Here's how the part is built. I have some questions about the finished solid (model axes, mm). A direction names the side the tool comes from. Give positions to 0.01 mm unless a question says otherwise; leave off trailing zeros. Order: outer loops, then holes, each group sorted by start corner. A loop starts at its lowest first (then second) coordinate and runs counter-clockwise, first axis right, second up.
from build123d import *

# Parameters (mm, degrees)
SKETCH1_R                  = 6
BOSS_EXTRUDE1_DEPTH        = 22
SKETCH2_R                  = 6
BOSS_EXTRUDE2_DEPTH        = 10
BOSS_EXTRUDE3_START        = -8
SKETCH3_R                  = 6
BOSS_EXTRUDE3_DEPTH        = 8
M6X1_0_TAPPED_HOLE1_D      = 5
M6X1_0_TAPPED_HOLE1_DEPTH  = 16
M6X1_0_TAPPED_HOLE1_TIP    = 1.443375673
SKETCH6_R                  = 6
CUT_EXTRUDE1_DEPTH         = 4
M6X1_0_TAPPED_HOLE2_REACH  = 63.741
M6X1_0_TAPPED_HOLE2_BORE_R = 2.5


with BuildPart() as part:
    # Sketch1 → Boss-Extrude1 (new body)
    with BuildSketch(Plane.XY):
        with BuildLine():
            Line((-8, 0), (8, 0))
            Line((8, 0), (8, 10))
            Line((8, 10), (32, 10))
            Line((32, 10), (32, 20))
            Line((32, 20), (24.228334067, 20))
            ThreePointArc((24.228334067, 20), (22.616435242, 20.469825663), (21.509410706, 21.732145215))
            Line((21.509410706, 21.732145215), (14.500924593, 36.761892188))
            ThreePointArc((14.500924593, 36.761892188), (0, 46), (-14.500924593, 36.761892188))
            Line((-14.500924593, 36.761892188), (-21.509410706, 21.732145215))
            ThreePointArc((-21.509410706, 21.732145215), (-22.616435242, 20.469825663), (-24.228334067, 20))
            Line((-24.228334067, 20), (-32, 20))
            Line((-32, 20), (-32, 10))
            Line((-32, 10), (-8, 10))
            Line((-8, 10), (-8, 0))
        make_face()
        with Locations((0, 30)):
            Circle(SKETCH1_R, mode=Mode.SUBTRACT)
    extrude(amount=-BOSS_EXTRUDE1_DEPTH)

    # Sketch2 → Boss-Extrude2 (add)
    with BuildSketch(Plane(origin=(0, 0, -22), x_dir=(-1, 0, 0), z_dir=(0, 0, -1))):
        Polygon((-32, 10), (-32, 46), (32, 46), (32, 10), (8, 10), (8, 0), (-8, 0), (-8, 10), align=None)
        with Locations(Location((0, 30, 0), (0, 0, 180))):
            Circle(SKETCH2_R, mode=Mode.SUBTRACT)
    extrude(amount=BOSS_EXTRUDE2_DEPTH)

    # Sketch3 → Boss-Extrude3 (add)
    with BuildSketch(Plane(origin=(0, 0, -32), x_dir=(-1, 0, 0), z_dir=(0, 0, -1)).offset(BOSS_EXTRUDE3_START)):
        with Locations(Location((0, 30, 0), (0, 0, 180))):
            Circle(SKETCH3_R)
    extrude(amount=BOSS_EXTRUDE3_DEPTH)

    # M6x1.0 Tapped Hole1
    with Locations(Plane(origin=(0, 0, 0), x_dir=(-1, 0, 0), z_dir=(0, -1, 0))):
        with Locations((0, 8), (0, 24)):
            Hole(M6X1_0_TAPPED_HOLE1_D / 2, depth=M6X1_0_TAPPED_HOLE1_DEPTH)
            with Locations((0, 0, -(M6X1_0_TAPPED_HOLE1_DEPTH + M6X1_0_TAPPED_HOLE1_TIP / 2))):  # 120° drill point
                Cone(0, M6X1_0_TAPPED_HOLE1_D / 2, M6X1_0_TAPPED_HOLE1_TIP, mode=Mode.SUBTRACT)

    # Sketch6 → Cut-Extrude1 (cut)
    with BuildSketch(Plane(origin=(0, 42, 0), x_dir=(1, 0, 0), z_dir=(0, 1, 0))):
        with Locations(Location((0, 12, 0), (0, 0, 90))):
            Circle(SKETCH6_R)
    extrude(amount=CUT_EXTRUDE1_DEPTH, mode=Mode.SUBTRACT)

    # M6x1.0 Tapped Hole2 bore → M6x1.0 Tapped Hole2 (cut, up to next)
    with BuildSketch(Plane(origin=(0, 42, 0), x_dir=(1, 0, 0), z_dir=(0, 1, 0)), mode=Mode.PRIVATE) as m6x1_0_tapped_hole2_sk1:
        with Locations((0, 12)):
            Circle(M6X1_0_TAPPED_HOLE2_BORE_R)
    m6x1_0_tapped_hole2_tool1 = extrude(m6x1_0_tapped_hole2_sk1.sketch, amount=-M6X1_0_TAPPED_HOLE2_REACH, mode=Mode.PRIVATE) & part.part
    add(m6x1_0_tapped_hole2_tool1.solids().sort_by_distance((0, 42, -12))[0], mode=Mode.SUBTRACT)


solid = part.part
Q1. If we section it at B-B on y = 14: List the corners of the cut face in (x, z) for me.
Filled sheet:
outline: (-32, -32) - (32, -32) - (32, 0) - (-32, 0) - close; hole circle Ø5 at (0, -24); hole circle Ø5 at (0, -8)
Q2. Thinking about a two-plate mould opening in Z: for faces 4 (the face through (0, 23, 0)), 5 (the face through (0, 0, -16)), 6 (the face through (-0.33, 38.77, -14.48)), which applies, released by +Z, released by -Z, zero draft, split by the parting line, or undercut?
Filled sheet:
face 4: released by +Z
face 5: zero draft
face 6: undercut
Q3. For faces 1 (the face through (22.637, 20.457, -10.846)), 2 (the face through (-0.33, 8.11, -26.48)), 3 (the face through (-23, 36, -22)), which set-ups out of +Z, -Z, +X, -X, +Y, -Y let a thin tool reach every point of the face, with its end or its side?
Filled sheet:
face 1: +Z, +X, +Y
face 2: -Y
face 3: +Z, -X, +Y
Q4. I need wall thicknesses on L1, parallel to Z at x = 0, y = 12.25; L2, parallel to X at y = 6.75, z = -24; L3, parallel to Y at x = 22, z = -23.5. Which ranges of each line are inside material? Lowest first, please.
Filled sheet:
L1: z = -32 to -26.5, -21.5 to -10.5, -5.5 to 0
L2: x = -8 to -2.5, 2.5 to 8
L3: y = 10 to 46
Q5. If we section it at A-A on z = -4: List the corners of the cut face in (x, y) for me, plus the area to 3 significant figures.
Filled sheet:
outline: (-32, 10) - (-8, 10) - (-8, 0) - (8, 0) - (8, 10) - (32, 10) - (32, 20) - (24.23, 20) arc R3 cw to (21.51, 21.73) - (14.5, 36.76) arc R16 ccw to (-14.5, 36.76) - (-21.51, 21.73) arc R3 cw to (-24.23, 20) - (-32, 20) - close; hole circle Ø12 at (0, 30)
area: 1,500 mm2
Q6. If we section it at C-C on z = -28: List the corners of the cut face in (x, y) for me, plus the area to 3 significant figures.
Filled sheet:
outline: (-32, 10) - (-8, 10) - (-8, 0) - (8, 0) - (8, 10) - (32, 10) - (32, 46) - (-32, 46) - close
area: 2,460 mm2
Q7. If we section it at D-D on x = 26: List the corners of the cut face in (y, z) for me.
Filled sheet:
outline: (10, -32) - (46, -32) - (46, -22) - (20, -22) - (20, 0) - (10, 0) - close
Q8. I'm going to push flat-ended pins straight in: P1, Ø8.5, axis at x = -28.5, z = -15, coming from the +Y side; P2, Ø19, axis at x = 0, y = 30, coming from the +Z side; P3, Ø3.5, axis at x = -1.5, z = -12, coming from the +Y side; P4, Ø2, axis at y = 22, z = -13, coming from the -X side. Where does each tip first touch, or does it pass through?
Filled sheet:
P1: stops at y = 20
P2: stops at z = 0
P3: stops at y = 42
P4: stops at x = -21.99
